The listing builds one solid part. Answer for the finished solid, in the listing's coordinates (mm). A direction names the side the tool comes from. Give positions to 0.01 mm unless a question says otherwise; leave off trailing zeros. Write each loop counter-clockwise with the first axis right and the second up, starting at its lowest first coordinate (ties: lowest second). Pieces come first, ordered by that corner, then holes. Notation, with made-up numbers: (62, -25.75) - (98, -25.75) arc R18 cw to (98, -13.75) - close; hole circle Ø2 at (73.25, 58.5). An arc over 180 degrees is marked (long way). Use a Markdown table: item, result. Add a question column.
from build123d import *

# Parameters (mm, degrees)
SKETCH1_R           = 15
SKETCH1_R_2         = 16
BOSS_EXTRUDE2_DEPTH = 16
SCALE1_SCALE        = 0.1
SKETCH2_W           = 8.2
SKETCH2_H           = 6
BOSS_EXTRUDE3_DEPTH = 2.2
CUT_EXTRUDE1_REACH  = 32.213
SKETCH3_R           = 0.6


with BuildPart() as part:
    # Sketch1 → Boss-Extrude2 (new body)
    with BuildSketch(Plane(origin=(0, 0, 0), x_dir=(1, 0, 0), z_dir=(0, 1, 0))):
        with BuildLine():
            Line((71.949541284, -40.775229358), (158.449541284, -40.775229358))
            ThreePointArc((158.449541284, -40.775229358), (218.449541284, 19.224770642), (158.449541284, 79.224770642))
            Line((158.449541284, 79.224770642), (-126.550458716, 79.224770642))
            ThreePointArc((-126.550458716, 79.224770642), (-168.976865587, 61.651177513), (-186.550458716, 19.224770642))
            Line((-186.550458716, 19.224770642), (-186.550458716, -40.775229358))
            Line((-186.550458716, -40.775229358), (-186.550458716, -69.775229358))
            ThreePointArc((-186.550458716, -69.775229358), (-155.550458716, -100.775229358), (-124.550458716, -69.775229358))
            Line((-124.550458716, -69.775229358), (-124.550458716, -69.275229358))
            ThreePointArc((-124.550458716, -69.275229358), (-116.203001979, -49.122686094), (-96.050458716, -40.775229358))
            Line((-96.050458716, -40.775229358), (-9.050458716, -40.775229358))
            ThreePointArc((-9.050458716, -40.775229358), (31.449541284, -0.275229358), (71.949541284, -40.775229358))
        make_face()
        with Locations(Location((158.449541284, 19.224770642, 0), (0, 0, 270))):
            Circle(SKETCH1_R, mode=Mode.SUBTRACT)
        with Locations(Location((-155.550458716, -38.775229358, 0), (0, 0, 270))):
            Circle(SKETCH1_R_2, mode=Mode.SUBTRACT)
    extrude(amount=BOSS_EXTRUDE2_DEPTH)


with BuildPart() as part_1:
    # Scale1: scaled about (-0.239262204, 8, -15.310747356)
    add(part.part.scale(SCALE1_SCALE).moved(Location((-0.215335984, 7.2, -13.77967262))))

    # Sketch2 → Boss-Extrude3 (add)
    with BuildSketch(Plane(origin=(0, 8.8, 0), x_dir=(1, 0, 0), z_dir=(0, 1, 0))):
        with Locations((-8.770381855, 18.702149685)):
            Rectangle(SKETCH2_W, SKETCH2_H)
    extrude(amount=BOSS_EXTRUDE3_DEPTH)

    # Sketch3 → Cut-Extrude1 (cut, up to next)
    with BuildSketch(Plane(origin=(0, 0, -21.702149685), x_dir=(-1, 0, 0), z_dir=(0, 0, -1)), mode=Mode.PRIVATE) as cut_extrude1_sk1:
        with Locations((6.670381855, 9.9)):
            Circle(SKETCH3_R)
    cut_extrude1_tool1 = extrude(cut_extrude1_sk1.sketch, amount=-CUT_EXTRUDE1_REACH, mode=Mode.PRIVATE) & part_1.part
    # Sketch3 → Cut-Extrude1 (cut, up to next)
    with BuildSketch(Plane(origin=(0, 0, -21.702149685), x_dir=(-1, 0, 0), z_dir=(0, 0, -1)), mode=Mode.PRIVATE) as cut_extrude1_sk2:
        with Locations((10.870381855, 9.9)):
            Circle(SKETCH3_R)
    cut_extrude1_tool2 = extrude(cut_extrude1_sk2.sketch, amount=-CUT_EXTRUDE1_REACH, mode=Mode.PRIVATE) & part_1.part
    add(cut_extrude1_tool1.solids().sort_by_distance((-6.670382, 9.9, -21.70215))[0], mode=Mode.SUBTRACT)
    add(cut_extrude1_tool2.solids().sort_by_distance((-10.870382, 9.9, -21.70215))[0], mode=Mode.SUBTRACT)


solid = part_1.part
1. Consider L1, parallel to X at y = 10, z = -18.25; L2, parallel to Z at x = 12.5, y = 8.35; L3, parallel to Y at x = 8.5, z = -18.5. Determine where each line is inside the solid, lowest interval first. Write a range as [from, to].
2. Given P1, Ø1.3, axis at x = 12, y = 8, coming from the +Z side; P2, Ø2.5, axis at x = -15.77, z = -9.9, coming from the +Y side; P3, Ø1.5, axis at x = 17, y = 9, coming from the -Z side; P4, Ø1.8, axis at y = 9.5, z = -19, coming from the +X side, each flat-ended and moving along its own axis, determine where each tip first touches the part or whether it passes through.
3. The part is cut by section D-D (x = 9). Give the vertices of the cut face in (y, z), and give its area (3 significant figures).
4. For a pull along X with two mould halves and no side action, classify faces 4 (the cylindrical face through (2.84, 7.99, -13.75)), 5 (the flat face through (-18.87, 8, -11)), 6 (the flat face through (-6, 8, -9.702)), 7 (the flat face through (-4.67, 10, -19)) as released by +X, released by -X, zero draft, split by the parting line, or undercut.
5. The part is cut by section C-C (z = -11). Give the vertices of the cut face in (x, y), and give its area (3 significant figures).
6. Which of the six approach directions +Z, -Z, +X, -X, +Y, -Y give full straight-line access (tool end or side, diameter ignored) to faces 1 (the flat face through (11, 8, -9.702)), 2 (the flat face through (-12.87, 10, -19)), 3 (the flat face through (-9, 10, -15.702))?
7. The part is cut by section B-B (z = -8.75). Give the vertices of the cut face in (x, y), and give its area (3 significant figures).
8. The part is cut by section A-A (y = 9.9). Give the vertices of the cut face in (x, z), and give its area (3 significant figures).
Check values:
| question | item | result |
|---|---|---|
| 1 | L1 | x = [-12.87, -11.46], [-10.28, -7.26], [-6.08, -4.67] |
| 1 | L2 | z = [-21.7, -9.7] |
| 1 | L3 | y = [7.2, 8.8] |
| 2 | P1 | stops at z = -9.7 |
| 2 | P2 | passes through |
| 2 | P3 | stops at z = -21.67 |
| 2 | P4 | stops at x = 20.97 |
| 3 | outline | (7.2, -21.7) - (8.8, -21.7) - (8.8, -9.7) - (7.2, -9.7) - close |
| 3 | area | 19.2 mm2 |
| 4 | face 4 | undercut |
| 4 | face 5 | released by -X |
| 4 | face 6 | zero draft |
| 4 | face 7 | released by +X |
| 5 | outline | (-18.87, 7.2) - (-16.93, 7.2) - (-16.93, 8.8) - (-18.87, 8.8) - close; (-14.61, 7.2) - (-0.91, 7.2) - (-0.91, 8.8) - (-14.61, 8.8) - close; (6.77, 7.2) - (19.36, 7.2) - (19.36, 8.8) - (6.77, 8.8) - close |
| 5 | area | 45.2 mm2 |
| 6 | face 1 | +Z, +X, +Y, -Y |
| 6 | face 2 | +Z, -Z, -X, +Y |
| 6 | face 3 | +Z, +X, -X, +Y |
| 7 | outline | (-18.87, 7.2) - (-16.88, 7.2) - (-16.88, 8.8) - (-18.87, 8.8) - close; (-14.66, 7.2) - (-11.95, 7.2) - (-11.95, 8.8) - (-14.66, 8.8) - close |
| 7 | area | 7.53 mm2 |
| 8 | outline | (-12.87, -21.7) - (-11.47, -21.7) - (-11.47, -15.7) - (-12.87, -15.7) - close; (-10.27, -21.7) - (-7.27, -21.7) - (-7.27, -15.7) - (-10.27, -15.7) - close; (-6.07, -21.7) - (-4.67, -21.7) - (-4.67, -15.7) - (-6.07, -15.7) - close |
| 8 | area | 34.8 mm2 |
